Here's the drawing with two shaded views (mm, measured from the low corner). I have some questions. A direction names the side the tool comes from. Give positions to 0.01 mm unless a question says otherwise; leave off trailing zeros. Order: outer loops, then holes, each group sorted by start corner. A loop starts at its lowest first (then second) coordinate and runs counter-clockwise, first axis right, second up. Notation, with made-up numbers: M 77,4.5 L 133,4.5 A33 cw 133,33.5 Z; hole C 5,80.5 d1. An arc over 180 degrees is marked long. Use a Markdown table: item, result. Add a question column.
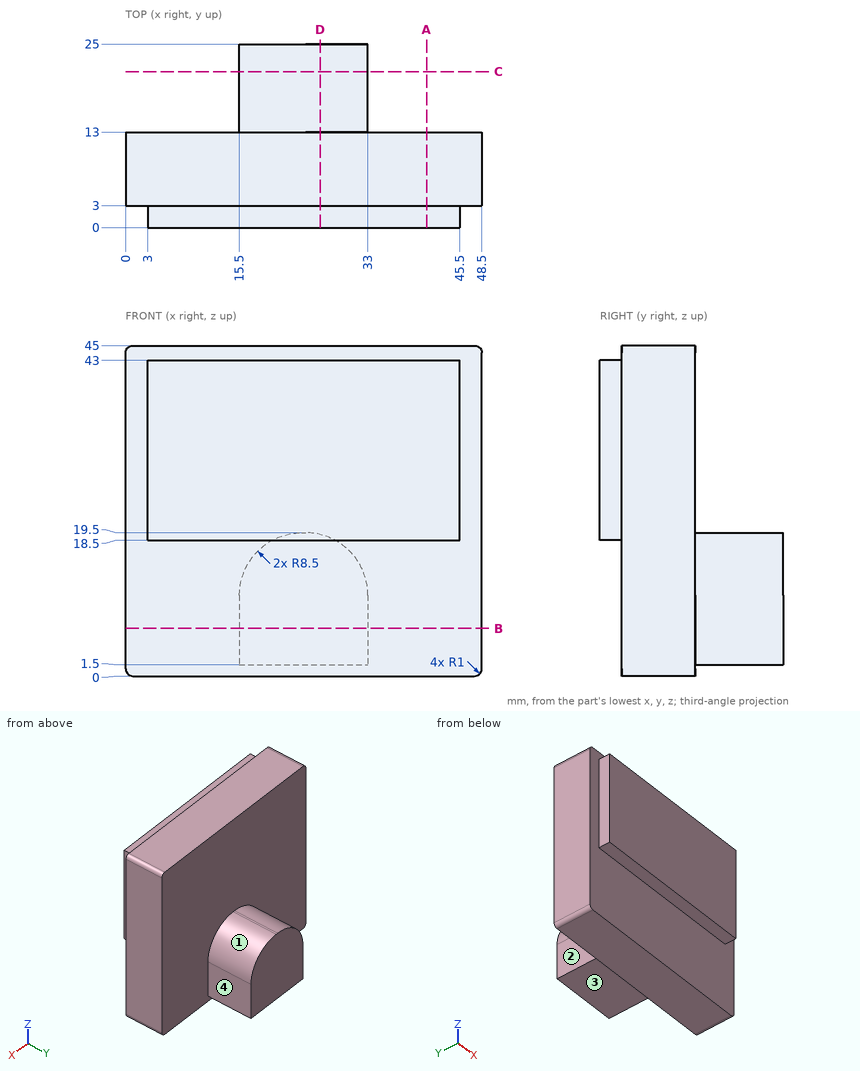
1. If we section it at D-D, the plane x = 26.5: List the corners of the cut face in (y, z) for me.
2. On a 3-axis mill with a long thin cutter (end or side, diameter ignored), from which of +Z, -Z, +X, -X, +Y, -Y can I reach the whole of each face in a straight line? I mean the marked faces 1, 2, 3 and 4. Say none if no direction works.
3. If we section it at C-C, the plane y = 21.25: List the corners of the cut face in (x, z) for me, then the cut area to 3 significant figures.
4. Will these pins go through, and if not, where does the flat tip stop? pin 1 (6 mm diameter, centred on y = 11, z = 30, fed in from -X); pin 2 (8 mm diameter, centred on y = 20.5, z = 6.5, fed in from +X); pin 3 (0.9 mm diameter, centred on y = 1, z = 31.5, fed in from -X); pin 4 (2.5 mm diameter, centred on x = 25.5, y = 1, fed in from -Z).
5. I need wall thicknesses on L1, parallel to Y at x = 30, z = 5; L2, parallel to Y at x = 4, z = 24.5; L3, parallel to Z at x = 37, y = 1.5. Which ranges of each line are inside material? Lowest first, please. Write a range as [from, to].
6. If we section it at A-A, the plane x = 41: List the corners of the cut face in (y, z) for me.
7. If we section it at B-B, the plane z = 6.5: List the corners of the cut face in (x, y) for me.
Geometry results:
| question | item | result |
|---|---|---|
| 1 | outline | M 0,18.5 L 3,18.5 L 3,0 L 13,0 L 13,1.5 L 25,1.5 L 25,19.26 L 13,19.26 L 13,45 L 3,45 L 3,43 L 0,43 Z |
| 2 | face 1 | +Z, +X, +Y |
| 2 | face 2 | +Z, -Z, -X, +Y |
| 2 | face 3 | -Z, +X, -X, +Y |
| 2 | face 4 | +Z, -Z, +X, +Y |
| 3 | outline | M 15.5,1.5 L 33,1.5 L 33,11 A8.5 ccw 24.5,19.5 L 24,19.5 A8.5 ccw 15.5,11 Z |
| 3 | area | 284 mm^2 |
| 4 | pin 1 | stops at x = 0 |
| 4 | pin 2 | stops at x = 33 |
| 4 | pin 3 | stops at x = 3 |
| 4 | pin 4 | stops at z = 18.5 |
| 5 | L1 | y = [3, 25] |
| 5 | L2 | y = [0, 13] |
| 5 | L3 | z = [18.5, 43] |
| 6 | outline | M 0,18.5 L 3,18.5 L 3,0 L 13,0 L 13,45 L 3,45 L 3,43 L 0,43 Z |
| 7 | outline | M 0,3 L 48.5,3 L 48.5,13 L 33,13 L 33,25 L 15.5,25 L 15.5,13 L 0,13 Z |
